Solid Edge part; units mm, degrees
sketch "Sketch1" plane through (0, 0, 0) normal (0, 0, 1) x (1, 0, 0)
  line L0 (0, 105) -> (0, 242)
  line L1 (0, 242) -> (-200, 242)
  line L2 (-200, 242) -> (-200, 122)
  line L3 (-200, 122) -> (-185, 122)
  line L4 (-185, 122) -> (-185, 107)
  line L5 (-185, 107) -> (-200, 107)
  line L6 (-200, 107) -> (-200, 0)
  line L7 (-200, 0) -> (-105, 0)
  arc A0 (-105, 0) -> (0, 105) centre (0, 0) cw
extrude "ProtrusiónExtruida_1" add sketch "Sketch1" along normal blind 40
fillet "Round1" radius 4 5 edges at (-105, 0, 20) (-200, 0, 20) (0, 105, 20) (0, 242, 20) (-200, 242, 20)
shell "Espesor_2" thickness 1.5 removed faces 1 at (-168.6667, 42.7533, 0)
sketch "Sketch2" plane through (-100, 121, 40) normal (0, 0, 1) x (1, 0, 0)
  line L0 (-19.8, -121) -> (-17.8, -121)
  arc A0 (-17.8, -121) -> (100, -3.2) centre (100, -121) cw
  line L1 (100, -3.2) -> (100, -1.2)
  arc A1 (-19.8, -121) -> (100, -1.2) centre (100, -121) cw
extrude "ProtrusiónExtruida_2" add sketch "Sketch2" along normal blind 0.01
sketch "Sketch3" plane through (-100, 121, 0) normal (0, 0, -1) x (-1, 0, 0)
  line L0 (77.5, -14) -> (77.5, 8.5)
  line L1 (77.5, 8.5) -> (100, 8.5)
  line L2 (100, 8.5) -> (100, -14)
  line L3 (100, -14) -> (77.5, -14)
extrude "VaciadoExtruido_1" cut sketch "Sketch3" against normal blind 4
Check sheet for the modelled part. Datum: model origin and axes. Units: mm. A direction names the side the tool comes from. Round coordinates to 2 decimals unless told otherwise and drop trailing zeros. Order: outer loops, then holes, each group sorted by start corner. A loop starts at its lowest first (then second) coordinate and runs counter-clockwise, first axis right, second up.
Q1. Set-up check for faces 1 (the face through (-153, 0, 20)), 2 (the face through (-99, 240.5, 19)): record each of +Z, -Z, +X, -X, +Y, -Y from which the full face is reachable in a straight line by a thin tool's end or side.
Filled sheet:
face 1: +Z, -Z, +X, -X, -Y
face 2: -Z
Q2. Cross-section at A-A, the plane z = 27.5. Enter the section's corners in (x, y).
Filled sheet:
outline: (-200, 4) arc R4 ccw to (-196, 0) - (-108.93, 0) arc R4 ccw to (-104.93, 3.85) arc R105 cw to (-3.85, 104.93) arc R4 ccw to (0, 108.93) - (0, 238) arc R4 ccw to (-4, 242) - (-196, 242) arc R4 ccw to (-200, 238) - (-200, 122) - (-185, 122) - (-185, 107) - (-200, 107) - close; hole (-198.5, 4) arc R2.5 ccw to (-196, 1.5) - (-108.93, 1.5) arc R2.5 ccw to (-106.43, 3.91) arc R106.5 cw to (-3.91, 106.43) arc R2.5 ccw to (-1.5, 108.93) - (-1.5, 238) arc R2.5 ccw to (-4, 240.5) - (-196, 240.5) arc R2.5 ccw to (-198.5, 238) - (-198.5, 123.5) - (-183.5, 123.5) - (-183.5, 105.5) - (-198.5, 105.5) - close
Q3. Cross-section at B-B, the plane x = -173.5. Enter the section's corners in (y, z), plus the area to 4 significant figures.
Filled sheet:
outline: (0, 0) - (1.5, 0) - (1.5, 38.5) - (240.5, 38.5) - (240.5, 0) - (242, 0) - (242, 40) - (0, 40) - close
area: 478.5 mm2
Q4. Draft check along X on faces 3 (the face through (-123, 149, 38.5)), 4 (the face through (-192, 107, 20)), 5 (the face through (-200, 56, 20)). Enter one of: pulls with the +X half, pulls with the -X half, needs draft (parallel to the pull), parting line crosses it, or undercut.
Filled sheet:
face 3: undercut
face 4: needs draft
face 5: pulls with the -X half
Q5. Cross-section at C-C, the plane y = 215.5. Enter the section's corners in (x, z), plus the area to 4 significant figures.
Filled sheet:
outline: (-200, 0) - (-198.5, 0) - (-198.5, 38.5) - (-1.5, 38.5) - (-1.5, 0) - (0, 0) - (0, 40) - (-200, 40) - close
area: 415.5 mm2
Q6. Scan lines: L1, parallel to Y at x = -158, z = 25; L2, parallel to X at y = 229, z = 32; L3, parallel to X at y = 113.5, z = 12. Record each from-to range of solid material in increasing order.
Filled sheet:
L1: y = 0 to 1.5, 240.5 to 242
L2: x = -200 to -198.5, -1.5 to 0
L3: x = -185 to -183.5, -1.5 to 0
Q7. Depth check by flat-ended pin: P1, Ø4, axis at x = -128.5, z = 28.5, coming from the -Y side; P2, Ø1, axis at x = -124, y = 62.5, coming from the -Z side; P3, Ø8, axis at x = -45, z = 11.5, coming from the -Y side; P4, Ø3, axis at y = 73, z = 10.5, coming from the +X side. Enter the tip coordinate at first touch or a pass-through.
Filled sheet:
P1: stops at y = 0
P2: stops at z = 38.5
P3: stops at y = 92.87
P4: stops at x = -73.99
